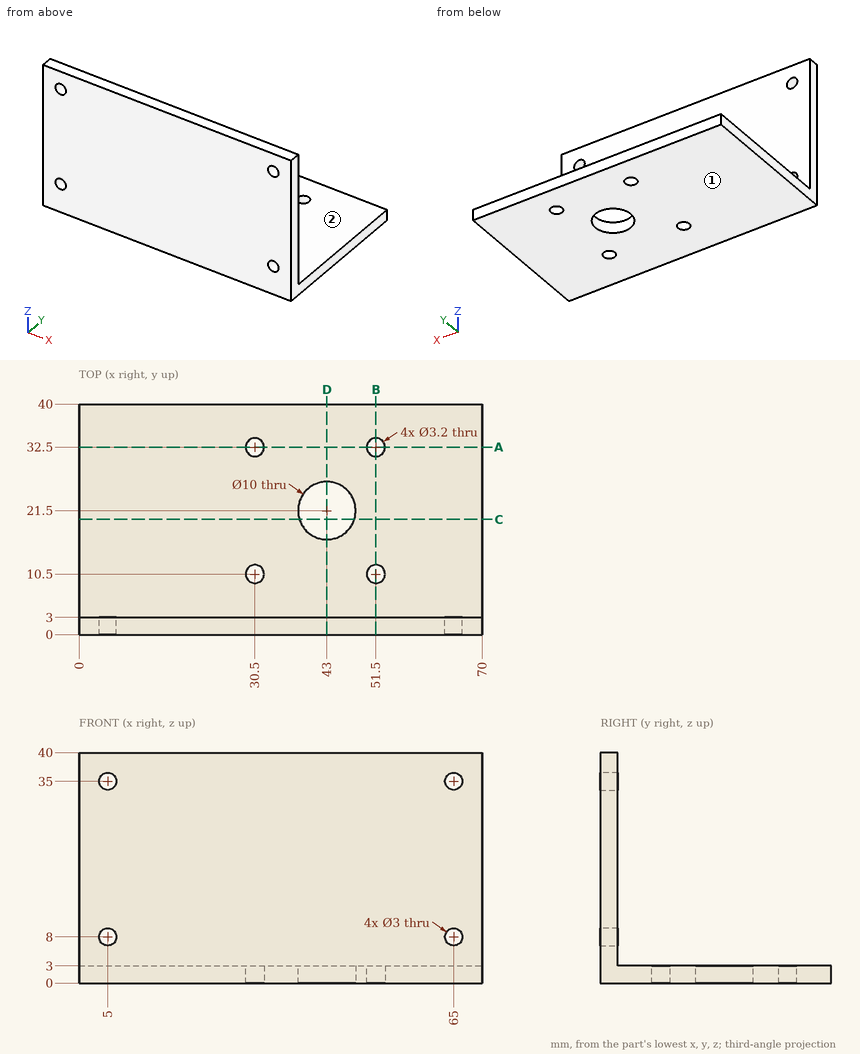
Answer from the drawing. Dimensions are ordinates in mm from the lowest x, y and z of the part. A direction names the side the tool comes from. Coordinates: 2 decimals unless noted, no trailing zeros. Loops run counter-clockwise (first coordinate to the right, second up) from the corner with the lowest first, then second, coordinate; pieces in that order, holes last.
1) Section B-B (x = 51.5) is taken. Give the vertices of the cut face in (y, z), plus the area to 3 significant figures.
Results:
outline: (0, 0) - (8.9, 0) - (8.9, 3) - (3, 3) - (3, 40) - (0, 40) - close; (12.1, 0) - (30.9, 0) - (30.9, 3) - (12.1, 3) - close; (34.1, 0) - (40, 0) - (40, 3) - (34.1, 3) - close
area: 212 mm2
2) Section A-A (y = 32.5) is taken. Give the vertices of the cut face in (x, z), plus the area to 3 significant figures.
Results:
outline: (0, 0) - (28.9, 0) - (28.9, 3) - (0, 3) - close; (32.1, 0) - (49.9, 0) - (49.9, 3) - (32.1, 3) - close; (53.1, 0) - (70, 0) - (70, 3) - (53.1, 3) - close
area: 191 mm2
3) Flat-ended cylindrical pins translate along their axes: pin 1 (2.5 mm diameter, centred on x = 5, z = 35, fed in from +Y); pin 2 (11 mm diameter, centred on x = 21.5, z = 16.5, fed in from +Y); pin 3 (3 mm diameter, centred on x = 62.5, y = 19, fed in from +Z). Find the tip coordinate at first contact, or state that the pin passes through.
Results:
pin 1: passes through
pin 2: stops at y = 3
pin 3: stops at z = 3
4) Section C-C (y = 20) is taken. Give the vertices of the cut face in (x, z), plus the area to 3 significant figures.
Results:
outline: (0, 0) - (38.23, 0) - (38.23, 3) - (0, 3) - close; (47.77, 0) - (70, 0) - (70, 3) - (47.77, 3) - close
area: 181 mm2
5) Section D-D (x = 43) is taken. Give the vertices of the cut face in (y, z).
Results:
outline: (0, 0) - (16.5, 0) - (16.5, 3) - (3, 3) - (3, 40) - (0, 40) - close; (26.5, 0) - (40, 0) - (40, 3) - (26.5, 3) - close
6) Consider probe 1 along Z at (x, y) = (65, 1); probe 2 along X at (y, z) = (2, 8); probe 3 along Y at (x, z) = (30, 1). Determine where each line is inside the solid, lowest interval first.
Results:
probe 1: z = 0 to 6.5, 9.5 to 33.5, 36.5 to 40
probe 2: x = 0 to 3.5, 6.5 to 63.5, 66.5 to 70
probe 3: y = 0 to 8.98, 12.02 to 30.98, 34.02 to 40
7) For the marked faces 1 and 2, determine the directions among +Z, -Z, +X, -X, +Y, -Y from which every point of the face is accessible in a straight line to the end or side of a thin tool.
Results:
face 1: -Z, +X, -X, +Y, -Y
face 2: +Z, +X, -X, +Y
